from build123d import *

# Parameters (mm, degrees)
BOSS_EXTRUDE1_DEPTH = 2
BOSS_EXTRUDE2_DEPTH = 8
SKETCH24_R          = 3.9
BOSS_EXTRUDE5_DEPTH = 4.4
SKETCH30_W          = 4.40861202
SKETCH30_H          = 1.324178481
CUT_EXTRUDE12_DEPTH = 16
CUT_EXTRUDE11_DEPTH = 23.928148639
FILLET1_R           = 1.5
SKETCH34_W          = 1.5
SKETCH34_H          = 1.5
CUT_EXTRUDE13_DEPTH = 8
SKETCH36_R          = 0.95
CUT_EXTRUDE15_DEPTH = 8
SKETCH37_R          = 2
CUT_EXTRUDE16_DEPTH = 4.5
SKETCH38_W          = 3
SKETCH38_H          = 1.25
CUT_EXTRUDE17_DEPTH = 3.6


with BuildPart() as part:
    # Sketch2 → Boss-Extrude1 (new body)
    with BuildSketch(Plane.XY):
        with BuildLine():
            Line((-2.5, 7.5), (-16.7, 7.5))
            Line((-16.7, 7.5), (-20.7, 3.793442666))
            Line((-20.7, 3.793442666), (-20.7, -4.031648778))
            Line((-20.7, -4.031648778), (-15.7, -7.5))
            Line((-15.7, -7.5), (-6.7, -7.5))
            Line((-6.7, -7.5), (-4.2, -5.6))
            ThreePointArc((-4.2, -5.6), (3.130495168, -6.260990337), (7, 0))
            ThreePointArc((7, 0), (4.949747468, 4.949747468), (0, 7))
            Line((0, 7), (0, 7.5))
            Line((0, 7.5), (-2.5, 7.5))
        make_face()
    extrude(amount=BOSS_EXTRUDE1_DEPTH)

    # Sketch4 → Boss-Extrude2 (add)
    with BuildSketch(Plane.XY.offset(2)):
        Polygon((-15.7, -7.5), (-6.7, -7.5), (-6.759079174, -4.5), (-7.7, -4.5), (-7.7, 2), (-5.5, 2), (-5.5, 5.3), (-2.5, 5.3), (-2.5, 7.5), (-16.7, 7.5), (-20.7, 3.793442666), (-20.7, -4.031648778), align=None)
    extrude(amount=BOSS_EXTRUDE2_DEPTH)

    # Sketch24 → Boss-Extrude5 (add)
    with BuildSketch(Plane.XY.offset(2)):
        Circle(SKETCH24_R)
    extrude(amount=BOSS_EXTRUDE5_DEPTH)

    # Sketch30 → Cut-Extrude12 (cut)
    with BuildSketch(Plane(origin=(-5.5, 0, 0), x_dir=(0, 0, -1), z_dir=(1, 0, 0))):
        with Locations((-4.20430601, 4.63791076)):
            Rectangle(SKETCH30_W, SKETCH30_H)
    extrude(amount=-CUT_EXTRUDE12_DEPTH, mode=Mode.SUBTRACT)

    # Sketch28 → Cut-Extrude11 (cut, through all)
    with BuildSketch(Plane.XY.offset(6.4)):
        with BuildLine():
            Line((-1, 0.979795897), (-1, -0.979795897))
            ThreePointArc((-1, -0.979795897), (1.4, 0), (-1, 0.979795897))
        make_face()
    extrude(amount=-CUT_EXTRUDE11_DEPTH, mode=Mode.SUBTRACT)

    # Fillet1
    # the kernel refuses this fillet: 1.5 mm, written as the material it takes off along each edge
    with BuildSketch(Plane(origin=(-15.230677435, -6, 1.5), x_dir=(-0.5699665637840448, -0.8216678867816415, 0), z_dir=(0, 0, -1))) as fillet1_piece_1_section:
        Polygon((0, 0), (FILLET1_R * 1.02, 0), (FILLET1_R * 1.02, -FILLET1_R * 0.319139344377), (FILLET1_R * 0.838101244517, -FILLET1_R * 0.58136589506), align=None)
    fillet1_piece_1 = extrude(amount=FILLET1_R * 1.02, mode=Mode.PRIVATE)
    fillet1_piece_1 = fillet1_piece_1 - Plane(origin=(-15.230677435, -6, 1.5), x_dir=(0.29860685961507855, 0.9543762064253388, 0), z_dir=(0, 0, -1)) * Sphere(FILLET1_R, mode=Mode.PRIVATE)
    add(fillet1_piece_1, mode=Mode.SUBTRACT)
    with BuildSketch(Plane(origin=(-16.11186344, 6, 1.5), x_dir=(-0.6796897201843015, 0.7334997506991983, 0), z_dir=(0, 0, -1))) as fillet1_piece_2_section:
        Polygon((0, 0), (FILLET1_R * 1.02, 0), (FILLET1_R * 1.02, FILLET1_R * 0.399932860855), (FILLET1_R * 0.748169745713, FILLET1_R * 0.693283514588), align=None)
    fillet1_piece_2 = extrude(amount=FILLET1_R * 1.02, mode=Mode.PRIVATE)
    fillet1_piece_2 = fillet1_piece_2 - Plane(origin=(-16.11186344, 6, 1.5), x_dir=(0.3650344157067945, -0.9309940254102596, 0), z_dir=(0, 0, -1)) * Sphere(FILLET1_R, mode=Mode.PRIVATE)
    add(fillet1_piece_2, mode=Mode.SUBTRACT)
    with BuildSketch(Plane(origin=(-19.2, 3.138411196, 1.5), x_dir=(-0.6796897201843015, 0.7334997506991983, 0), z_dir=(0, 0, -1))) as fillet1_piece_3_section:
        Polygon((0, 0), (FILLET1_R * 1.02, 0), (FILLET1_R * 1.02, -FILLET1_R * 0.445421399395), (FILLET1_R * 0.693283514588, -FILLET1_R * 0.748169745713), align=None)
    fillet1_piece_3 = extrude(amount=FILLET1_R * 1.02, mode=Mode.PRIVATE)
    fillet1_piece_3 = fillet1_piece_3 - Plane(origin=(-19.2, 3.138411196, 1.5), x_dir=(0.9164304993244992, -0.40019387789901173, 0), z_dir=(0, 0, -1)) * Sphere(FILLET1_R, mode=Mode.PRIVATE)
    add(fillet1_piece_3, mode=Mode.SUBTRACT)
    with BuildSketch(Plane(origin=(-19.2, -3.246599046, 1.5), x_dir=(-0.5699665637840448, -0.8216678867816415, 0), z_dir=(0, 0, -1))) as fillet1_piece_4_section:
        Polygon((0, 0), (FILLET1_R * 1.02, 0), (FILLET1_R * 1.02, FILLET1_R * 0.533833817771), (FILLET1_R * 0.58136589506, FILLET1_R * 0.838101244517), align=None)
    fillet1_piece_4 = extrude(amount=FILLET1_R * 1.02, mode=Mode.PRIVATE)
    fillet1_piece_4 = fillet1_piece_4 - Plane(origin=(-19.2, -3.246599046, 1.5), x_dir=(0.8859928227090906, 0.46369895202380795, 0), z_dir=(0, 0, -1)) * Sphere(FILLET1_R, mode=Mode.PRIVATE)
    add(fillet1_piece_4, mode=Mode.SUBTRACT)
    with BuildSketch(Plane(origin=(-15.230677435, -7.5, 0), x_dir=(0, 1, 0), z_dir=(1, 0, 0))) as fillet1_piece_5_section:
        with BuildLine():
            CenterArc((FILLET1_R, FILLET1_R), FILLET1_R, 180, 90)
            Line((0, FILLET1_R), (0, 0))
            Line((0, 0), (FILLET1_R, 0))
        make_face()
    fillet1_piece_5 = extrude(amount=12.280677435, mode=Mode.PRIVATE)
    fillet1_piece_5 = split(fillet1_piece_5, bisect_by=Plane(origin=(-9.092127217, -9.318016685, 0.3282266), z_dir=(-0.6050832675335577, 0.7961621941231027, 0)), keep=Keep.TOP, mode=Mode.PRIVATE)
    add(fillet1_piece_5, mode=Mode.SUBTRACT)
    with BuildSketch(Plane(origin=(3.75, 7.5, 0), x_dir=(0, 0, 1), z_dir=(-1, 0, 0))) as fillet1_piece_6:
        with BuildLine():
            CenterArc((FILLET1_R, -FILLET1_R), FILLET1_R, 90, 90)
            Line((0, -FILLET1_R), (0, 0))
            Line((0, 0), (FILLET1_R, 0))
        make_face()
    extrude(amount=19.86186344, mode=Mode.SUBTRACT)
    with BuildSketch(Plane(origin=(-17.13139802, 7.100249626, 0), x_dir=(0.6796897201843014, -0.7334997506991981, 0), z_dir=(-0.7334997506991983, -0.6796897201843015, 0))) as fillet1_piece_7:
        with BuildLine():
            CenterArc((FILLET1_R, FILLET1_R), FILLET1_R, 180, 90)
            Line((0, FILLET1_R), (0, 0))
            Line((0, 0), (FILLET1_R, 0))
        make_face()
    extrude(amount=4.21013989, mode=Mode.SUBTRACT)
    with BuildSketch(Plane(origin=(-20.054949846, -4.479100876, 0), x_dir=(0.5699665637840448, 0.8216678867816416, 0), z_dir=(0.8216678867816415, -0.5699665637840448, 0))) as fillet1_piece_8:
        with BuildLine():
            CenterArc((FILLET1_R, FILLET1_R), FILLET1_R, 180, 90)
            Line((0, FILLET1_R), (0, 0))
            Line((0, 0), (FILLET1_R, 0))
        make_face()
    extrude(amount=4.830811364, mode=Mode.SUBTRACT)
    with BuildSketch(Plane(origin=(-20.7, 3.138411196, 0), x_dir=(1, 0, 0), z_dir=(0, -1, 0))) as fillet1_piece_9:
        with BuildLine():
            CenterArc((FILLET1_R, FILLET1_R), FILLET1_R, 180, 90)
            Line((0, FILLET1_R), (0, 0))
            Line((0, 0), (FILLET1_R, 0))
        make_face()
    extrude(amount=6.385010242, mode=Mode.SUBTRACT)
    with BuildSketch(Plane(origin=(-15.7, -7.5, 1.5), x_dir=(1, 0, 0), z_dir=(0, 0, 1))) as fillet1_piece_10:
        with BuildLine():
            CenterArc((FILLET1_R * 0.312881710173, FILLET1_R), FILLET1_R, 235.252105822, 34.747894178)
            Line((-FILLET1_R * 0.257084853611, FILLET1_R * 0.178332113218), (0, 0))
            Line((0, 0), (FILLET1_R * 0.312881710173, 0))
        make_face()
    extrude(amount=9.673306413, mode=Mode.SUBTRACT)
    with BuildSketch(Plane(origin=(-20.7, -4.031648778, 1.5), x_dir=(0, 1, 0), z_dir=(0, 0, 1))) as fillet1_piece_11:
        with BuildLine():
            CenterArc((FILLET1_R * 0.523366488011, -FILLET1_R), FILLET1_R, 90, 55.252105822)
            Line((-FILLET1_R * 0.298301398771, -FILLET1_R * 0.430033436216), (0, 0))
            Line((0, 0), (FILLET1_R * 0.523366488011, 0))
        make_face()
    extrude(amount=10.46262433, mode=Mode.SUBTRACT)
    with BuildSketch(Plane(origin=(-20.7, 3.793442666, 1.5), x_dir=(0.7334997506991984, 0.6796897201843014, 0), z_dir=(0, 0, 1))) as fillet1_piece_12:
        with BuildLine():
            CenterArc((FILLET1_R * 0.436687646465, -FILLET1_R), FILLET1_R, 90, 47.18059856)
            Line((-FILLET1_R * 0.296812104234, -FILLET1_R * 0.320310279816), (0, 0))
            Line((0, 0), (FILLET1_R * 0.436687646465, 0))
        make_face()
    extrude(amount=10.137578674, mode=Mode.SUBTRACT)
    with BuildSketch(Plane(origin=(-16.7, 7.5, 1.5), x_dir=(1, 0, 0), z_dir=(0, 0, 1))) as fillet1_piece_13:
        with BuildLine():
            CenterArc((FILLET1_R * 0.392091040054, -FILLET1_R), FILLET1_R, 90, 42.81940144)
            Line((-FILLET1_R * 0.287598680131, -FILLET1_R * 0.266500249301), (0, 0))
            Line((0, 0), (FILLET1_R * 0.392091040054, 0))
        make_face()
    extrude(amount=9.9703414, mode=Mode.SUBTRACT)

    # Sketch34 → Cut-Extrude13 (cut, along a direction that is not the sketch's normal)
    with BuildSketch(Plane.XZ.offset(-2)):
        with Locations((-6.95, 10)):
            Rectangle(SKETCH34_W, SKETCH34_H)
    extrude(amount=-CUT_EXTRUDE13_DEPTH, dir=(0.6685833876565112, -0.7436371788377336, 0), mode=Mode.SUBTRACT)

    # Sketch36 → Cut-Extrude15 (cut)
    with BuildSketch(Plane.XY.offset(10)):
        with Locations((-11.7, 0)):
            Circle(SKETCH36_R)
        with Locations((-16.7, 0)):
            Circle(SKETCH36_R)
    extrude(amount=-CUT_EXTRUDE15_DEPTH, mode=Mode.SUBTRACT)

    # Sketch37 → Cut-Extrude16 (cut)
    with BuildSketch(Plane(origin=(0, 0, 0), x_dir=(-1, 0, 0), z_dir=(0, 0, -1))):
        with Locations((11.7, 0)):
            Circle(SKETCH37_R)
        with Locations((16.7, 0)):
            Circle(SKETCH37_R)
    extrude(amount=-CUT_EXTRUDE16_DEPTH, mode=Mode.SUBTRACT)

    # Sketch38 → Cut-Extrude17 (cut)
    with BuildSketch(Plane.XY.offset(10)):
        with Locations((-4, 5.925)):
            Rectangle(SKETCH38_W, SKETCH38_H)
    extrude(amount=-CUT_EXTRUDE17_DEPTH, mode=Mode.SUBTRACT)


with BuildPart() as body_2:
    # Split1: the piece on the far side of the plane
    add(part.part)
    split(bisect_by=Plane.XY.offset(6.4), keep=Keep.BOTTOM)


with BuildPart() as part_1:
    add(part.part)

    # Split1
    split(bisect_by=Plane.XY.offset(6.4), keep=Keep.TOP)


solid = body_2.part
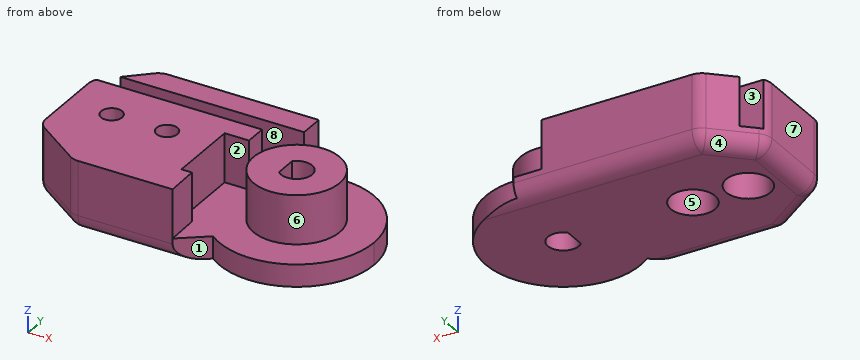
Can you work these out from the model? Positions are in its coordinate system, mm. Face numbers are marked on the shaded views. A direction names the side the tool comes from. Give positions to 0.01 mm unless a question says otherwise; leave off trailing zeros. Loops run counter-clockwise (first coordinate to the right, second up) from the corner with the lowest first, then second, coordinate; pieces in that order, holes last. Notation, with made-up numbers: (1.5, -4.5) - (50.5, -4.5) arc R19 ccw to (50.5, 17.5) - close; hole circle Ø10 at (-21.75, 63.25). An arc over 180 degrees is marked (long way). Answer as a JSON object with one key per item and string values.
Q1. Will these pins go through, and if not, where does the flat tip stop? P1, Ø3.5, axis at x = -11.7, y = 0, coming from the -Z side; P2, Ø1.5, axis at x = -11.7, y = 0, coming from the -Z side; P3, Ø1.8, axis at y = 6.5, z = 3, coming from the +X side; P4, Ø1, axis at x = 0.5, z = 4, coming from the +Y side.
Geometry says:
{"P1": "z = 4.5", "P2": "through", "P3": "x = -2.5", "P4": "y = 3.9"}
Q2. If we mould it in two halves opening along Y, with no side actions, what happens to the marked faces 1, 2, 3 and 4? For each: pulls with the +Y half, pulls with the -Y half, needs draft (parallel to the pull), parting line crosses it, or undercut.
Geometry says:
{"face 1": "pulls with the -Y half", "face 2": "undercut", "face 3": "undercut", "face 4": "pulls with the +Y half"}
Q3. Imagine slicing it at C-C on z = 5. Write out the boundary of the cut face in (x, y), plus the area to 3 significant figures.
Geometry says:
{"outline": "(-20.7, -3.25) arc R1.5 ccw to (-20.05, -4.48) - (-16.09, -7.23) arc R1.5 ccw to (-15.23, -7.5) - (-6.7, -7.5) - (-6.76, -4.5) - (-7.7, -4.5) - (-7.7, 2) - (-5.5, 2) - (-5.5, 3.98) - (-20.44, 3.98) arc R1.5 ccw to (-20.7, 3.14) - close; (-19.07, 5.3) - (-2.5, 5.3) - (-2.5, 7.5) - (-16.11, 7.5) arc R1.5 ccw to (-17.13, 7.1) - close; circle Ø7.8 at (0, 0); hole circle Ø1.9 at (-16.7, 0); hole circle Ø1.9 at (-11.7, 0); hole (-1, -0.98) arc R1.4 ccw (long way) to (-1, 0.98) - close", "area": "218 mm²"}
Q4. Imagine slicing it at D-D on y = 2.75. Write out the boundary of the cut face in (x, z).
Geometry says:
{"outline": "(-20.7, 1.5) arc R1.5 ccw to (-19.2, 0) - (6.44, 0) - (6.44, 2) - (2.77, 2) - (2.77, 6.4) - (-2.77, 6.4) - (-2.77, 2) - (-5.5, 2) - (-5.5, 6.4) - (-20.7, 6.4) - close"}
Q5. If I drill on L1, parallel to Y at x = -11.7, z = 5.55; L2, parallel to Y at x = -16, z = 3.5; L3, parallel to X at y = 1.5, z = 1.5, over which ranges is the centre line in solid material (lowest first)?
Geometry says:
{"L1": "-7.5 to -0.95, 0.95 to 3.98, 5.3 to 7.5", "L2": "-7.29 to -1.87, 1.87 to 3.98, 5.3 to 7.5", "L3": "-20.7 to -18.02, -15.38 to -13.02, -10.38 to 6.84"}
Q6. Which directions (+Z, -Z, +X, -X, +Y, -Y) give clear straight access to the entire face, cutting with the end or side of a thin tool? Please do the marked faces 5, 6, 7 and 8.
Geometry says:
{"face 5": "-Z", "face 6": "+Z", "face 7": "+Z, -Z, -X, +Y, -Y", "face 8": "+Z, +X, -X"}
Q7. Imagine slicing it at B-B on x = -11.7. Write out the boundary of the cut face in (y, z), plus the area to 3 significant figures.
Geometry says:
{"outline": "(-7.5, 1.5) arc R1.5 ccw to (-6, 0) - (-2, 0) - (-2, 4.5) - (-0.95, 4.5) - (-0.95, 6.4) - (-7.5, 6.4) - close; (0.95, 4.5) - (2, 4.5) - (2, 0) - (6, 0) arc R1.5 ccw to (7.5, 1.5) - (7.5, 6.4) - (5.3, 6.4) - (5.3, 2) - (3.98, 2) - (3.98, 6.4) - (0.95, 6.4) - close", "area": "67.6 mm²"}
Q8. Imagine slicing it at A-A on z = 3. Write out the boundary of the cut face in (x, y), plus the area to 3 significant figures.
Geometry says:
{"outline": "(-20.7, -3.25) arc R1.5 ccw to (-20.05, -4.48) - (-16.09, -7.23) arc R1.5 ccw to (-15.23, -7.5) - (-6.7, -7.5) - (-6.76, -4.5) - (-7.7, -4.5) - (-7.7, 2) - (-5.5, 2) - (-5.5, 3.98) - (-20.44, 3.98) arc R1.5 ccw to (-20.7, 3.14) - close; (-19.07, 5.3) - (-2.5, 5.3) - (-2.5, 7.5) - (-16.11, 7.5) arc R1.5 ccw to (-17.13, 7.1) - close; circle Ø7.8 at (0, 0); hole circle Ø4 at (-16.7, 0); hole circle Ø4 at (-11.7, 0); hole (-1, -0.98) arc R1.4 ccw (long way) to (-1, 0.98) - close", "area": "198 mm²"}
